from build123d import *

# Parameters (mm, degrees)
PAD_DEPTH       = 38.1
SKETCH001_R     = 50.8
SKETCH001_R_2   = 41.148
POCKET_DEPTH    = 38.101
SKETCH002_R     = 6.35
POCKET001_DEPTH = 50.801
POCKET002_DEPTH = 9.652


with BuildPart() as part:
    # Sketch → Pad (new body, symmetric)
    with BuildSketch(Plane.YZ):
        with BuildLine():
            ThreePointArc((-29.591, -41.2918), (0, -50.8), (29.591, -41.2918))
            Line((29.591, -41.2918), (22.352, 0))
            Line((22.352, 0), (-22.352, 0))
            Line((-29.591, -41.2918), (-22.352, 0))
        make_face()
    extrude(amount=PAD_DEPTH, both=True)

    # Sketch001 → Pocket (cut, through all)
    with BuildSketch(Plane.YZ):
        Circle(SKETCH001_R)
        Circle(SKETCH001_R_2, mode=Mode.SUBTRACT)
    extrude(amount=POCKET_DEPTH, mode=Mode.SUBTRACT)

    # Sketch002 → Pocket001 (cut, through all)
    with BuildSketch(Plane.XY):
        with Locations((-19.05, 0)):
            Circle(SKETCH002_R)
        with Locations((19.05, 0)):
            Circle(SKETCH002_R)
    extrude(amount=-POCKET001_DEPTH, mode=Mode.SUBTRACT)

    # Sketch003 → Pocket002 (cut)
    with BuildSketch(Plane.XY):
        Polygon((-26.924, 31.75), (-11.176, 31.75), (-11.176, 12.7), (38.1, 12.7), (38.1, -12.7), (-11.176, -12.7), (-11.176, -31.75), (-26.924, -31.75), (-26.924, -12.7), (-38.1, -12.7), (-38.1, 12.7), (-26.924, 12.7), align=None)
    extrude(amount=-POCKET002_DEPTH, mode=Mode.SUBTRACT)


solid = part.part
The model under review builds one solid part; all positions refer to its coordinate system, in mm. A direction names the side the tool comes from. Coordinates: 2 decimals unless noted, no trailing zeros. Write each loop counter-clockwise with the first axis right and the second up, starting at its lowest first coordinate (ties: lowest second). Pieces come first, ordered by that corner, then holes. Notation, with made-up numbers: M 74.5,21 L 123.5,21 A19 cw 123.5,46 Z; hole C -6,24 d1. An arc over 180 degrees is marked long. Put each result on its own line as item: value.
1) Wall thickness on probe 1 along X at (y, z) = (0, -30.5); probe 2 along X at (y, z) = (-21, -8.5); probe 3 along X at (y, z) = (-12, -45.5): over which ranges is each line inside the solid? List them lowest first. Write a range as [from, to].
Computed:
probe 1: x = [-38.1, -25.4], [-12.7, 12.7], [25.4, 38.1]
probe 2: x = [-38.1, -26.92], [-11.18, 38.1]
probe 3: x = [-38.1, 0]
2) Add section D-D on x = -19.05. Give the boundary of the cut face in (y, z).
Computed:
outline: M -29.59,-41.29 A50.8 ccw -6.35,-50.4 L -6.35,-9.65 L -24.04,-9.65 Z; M 6.35,-50.4 A50.8 ccw 29.59,-41.29 L 24.04,-9.65 L 6.35,-9.65 Z
3) Add section A-A on y = 0. Give the boundary of the cut face in (x, z), then the cut area to 3 significant figures.
Computed:
outline: M -38.1,-50.8 L -25.4,-50.8 L -25.4,-9.65 L -38.1,-9.65 Z; M -12.7,-50.8 L 0,-50.8 L 0,-41.15 L 12.7,-41.15 L 12.7,-9.65 L -12.7,-9.65 Z; M 25.4,-41.15 L 38.1,-41.15 L 38.1,-9.65 L 25.4,-9.65 Z
area: 1,850 mm2
4) For faces 4 (the flat face through (-32, 18, 0)), 5 (the flat face through (-11.176, -18, -5)), 6 (the cylindrical face through (18.783, -7.138, -40.524)), 7 (the flat face through (13, 12.7, -5)), list the 3-axis set-ups (+Z, -Z, +X, -X, +Y, -Y) from which the entire face can be reached by the end or side of a thin tool; tool diameter is ignored.
Computed:
face 4: +Z, +X, -X, +Y, -Y
face 5: +Z, +Y, -Y
face 6: -Z, +X
face 7: +Z, +X, -X
5) Clearance check with flat-ended pins moving along their axes: pin 1 Ø1.5 at (x, z) = (-8, -33.5) entering from +Y; pin 2 Ø5 at (x, z) = (-1.5, -33.5) entering from -Y; pin 3 Ø7.5 at (x, z) = (-33, -3) entering from -Y. State where each tip first meets the part, or that it passes through.
Computed:
pin 1: stops at y = 28.36
pin 2: stops at y = -28.66
pin 3: stops at y = -23.54
6) Add section B-B on x = 19.05. Give the boundary of the cut face in (y, z).
Computed:
outline: M -27.69,-30.44 A41.15 ccw -6.35,-40.66 L -6.35,-9.65 L -12.7,-9.65 L -12.7,0 L -22.35,0 Z; M 6.35,-40.66 A41.15 ccw 27.69,-30.44 L 22.35,0 L 12.7,0 L 12.7,-9.65 L 6.35,-9.65 Z
7) Add section C-C on y = 19. Give the boundary of the cut face in (x, z).
Computed:
outline: M -38.1,-47.11 L 0,-47.11 L 0,-36.5 L 38.1,-36.5 L 38.1,0 L -11.18,0 L -11.18,-9.65 L -26.92,-9.65 L -26.92,0 L -38.1,0 Z
8) Draft analysis for pull direction X (two halves, no side actions). For faces 1 (the cylindrical face through (-24.09, -3.86, -29.94)), 2 (the flat face through (-38.1, 0, -25)), 3 (the flat face through (-32, -12.7, -5)), state which applies: released by +X, released by -X, zero draft, split by the parting line, or undercut.
Computed:
face 1: undercut
face 2: released by -X
face 3: zero draft
